Work out the finished part from the listing and answer in its coordinate system (mm). A direction names the side the tool comes from. Give positions to 0.01 mm unless a question says otherwise; leave off trailing zeros. Order: outer loops, then holes, each group sorted by start corner. A loop starts at its lowest first (then second) coordinate and runs counter-clockwise, first axis right, second up. Notation, with made-up numbers: (7.5, 20.25) -> (57.5, 20.25) arc R34 cw to (57.5, 54.25) -> close; hole circle Ø11 at (-27, 74). An arc over 180 degrees is marked (long way). Use a Markdown table: item, result. Add a question column.
```python
from build123d import *

# Parameters (mm, degrees)
BASIC_SHAPE_SKETCH_R                = 49
BASIC_SHAPE_SKETCH_R_2              = 22.5
BASIC_SHAPE_DEPTH                   = 68.03
SLIT_DEPTH                          = 98.108603635
BATTERY_SLOT_SKETCH_R               = 9.65
BATTERY_SLOT_DEPTH                  = 67.03
PATTERN_BATTERY_SLOT_COUNT          = 5
PATTERN_BATTERY_SLOT_ANGLE          = 130.88
MIRROR_BATTERY_SLOT_COPY_1_SKETCH_R = 9.65
MIRROR_BATTERY_SLOT_COPY_1_DEPTH    = 67.03
MIRROR_BATTERY_SLOT_COPY_2_SKETCH_R = 9.65
MIRROR_BATTERY_SLOT_COPY_2_DEPTH    = 67.03
MIRROR_BATTERY_SLOT_COPY_3_SKETCH_R = 9.65
MIRROR_BATTERY_SLOT_COPY_3_DEPTH    = 67.03
MIRROR_BATTERY_SLOT_COPY_4_SKETCH_R = 9.65
MIRROR_BATTERY_SLOT_COPY_4_DEPTH    = 67.03
BUS_SLIT_DEPTH                      = 67.03
CAP_INNER_LIP_DEPTH                 = 4.8
CAP_OUTER_LIP_DEPTH                 = 4.8
WIRE_SLITS_DEPTH                    = 98.108603635
WIRE_SLITS_DEPTH_BACK               = 67.03
PENNY_HOLE_SKETCH_R                 = 9.65
PENNY_HOLE_DEPTH                    = 100.807559333


with BuildPart() as part:
    # Basic_Shape_Sketch → Basic_Shape (new body)
    with BuildSketch(Plane.XY):
        Circle(BASIC_SHAPE_SKETCH_R)
        Circle(BASIC_SHAPE_SKETCH_R_2, mode=Mode.SUBTRACT)
    extrude(amount=BASIC_SHAPE_DEPTH)

    # Slit_Sketch → Slit (cut, through all)
    with BuildSketch(Plane.XY.offset(68.03)):
        with BuildLine():
            Line((-8.33, 48.286759055), (-8.33, 20.901222452))
            Line((-8.33, 20.901222452), (8.33, 20.901222452))
            Line((8.33, 20.901222452), (8.33, 48.286759055))
            ThreePointArc((8.33, 48.286759055), (0, 56.616759055), (-8.33, 48.286759055))
        make_face()
    extrude(amount=-SLIT_DEPTH, mode=Mode.SUBTRACT)

    # Battery_Slot_Sketch → Battery_Slot (cut)
    with BuildSketch(Plane.XY.offset(68.03)):
        with Locations((-10.069761866, -34.302512969)):
            Circle(BATTERY_SLOT_SKETCH_R)
    battery_slot = extrude(amount=-BATTERY_SLOT_DEPTH, mode=Mode.SUBTRACT)

    # Pattern_Battery_Slot: Battery_Slot ×5 about axis
    pattern_battery_slot_axis = Axis((0, 0, 0), (0, 0, -1))
    for i in range(1, PATTERN_BATTERY_SLOT_COUNT):
        add(battery_slot.rotate(pattern_battery_slot_axis, i * PATTERN_BATTERY_SLOT_ANGLE / (PATTERN_BATTERY_SLOT_COUNT - 1)), mode=Mode.SUBTRACT)

    # Mirror_Battery_Slot: Battery_Slot across plane
    add(battery_slot.mirror(Plane(origin=(0, 0, 0), x_dir=(0, 0, 1), z_dir=(1, 0, 0))), mode=Mode.SUBTRACT)

    # Mirror_Battery_Slot copy 1 sketch → Mirror_Battery_Slot copy 1 (cut)
    with BuildSketch(Plane(origin=(0, 0, 68.03), x_dir=(-0.8413221512344797, -0.5405340302350882, 0), z_dir=(0, 0, 1))):
        with Locations((-10.069761866, 34.302512969)):
            Circle(MIRROR_BATTERY_SLOT_COPY_1_SKETCH_R)
    extrude(amount=-MIRROR_BATTERY_SLOT_COPY_1_DEPTH, mode=Mode.SUBTRACT)

    # Mirror_Battery_Slot copy 2 sketch → Mirror_Battery_Slot copy 2 (cut)
    with BuildSketch(Plane(origin=(0, 0, 68.03), x_dir=(-0.4156459243156256, -0.9095265062656553, 0), z_dir=(0, 0, 1))):
        with Locations((-10.069761866, 34.302512969)):
            Circle(MIRROR_BATTERY_SLOT_COPY_2_SKETCH_R)
    extrude(amount=-MIRROR_BATTERY_SLOT_COPY_2_DEPTH, mode=Mode.SUBTRACT)

    # Mirror_Battery_Slot copy 3 sketch → Mirror_Battery_Slot copy 3 (cut)
    with BuildSketch(Plane(origin=(0, 0, 68.03), x_dir=(0.14193790484034807, -0.9898755634773152, 0), z_dir=(0, 0, 1))):
        with Locations((-10.069761866, 34.302512969)):
            Circle(MIRROR_BATTERY_SLOT_COPY_3_SKETCH_R)
    extrude(amount=-MIRROR_BATTERY_SLOT_COPY_3_DEPTH, mode=Mode.SUBTRACT)

    # Mirror_Battery_Slot copy 4 sketch → Mirror_Battery_Slot copy 4 (cut)
    with BuildSketch(Plane(origin=(0, 0, 68.03), x_dir=(0.6544769311996185, -0.7560819707726999, 0), z_dir=(0, 0, 1))):
        with Locations((-10.069761866, 34.302512969)):
            Circle(MIRROR_BATTERY_SLOT_COPY_4_SKETCH_R)
    extrude(amount=-MIRROR_BATTERY_SLOT_COPY_4_DEPTH, mode=Mode.SUBTRACT)

    # Bus_Slit_Sketch → Bus_Slit (cut)
    with BuildSketch(Plane.XY.offset(68.03)):
        with BuildLine():
            ThreePointArc((-9.754463235, 31.132636766), (0, -32.625), (9.754463235, 31.132636766))
            ThreePointArc((9.754463235, 31.132636766), (10.629095474, 34.20551129), (12.459123069, 36.824392423))
            ThreePointArc((12.459123069, 36.824392423), (0, -38.875), (-12.459123069, 36.824392423))
            ThreePointArc((-12.459123069, 36.824392423), (-10.629095474, 34.20551129), (-9.754463235, 31.132636766))
        make_face()
    extrude(amount=-BUS_SLIT_DEPTH, mode=Mode.SUBTRACT)

    # Cap_Inner_Lip_Sketch → Cap_Inner_Lip (add)
    with BuildSketch(Plane.XY.offset(68.03)):
        with BuildLine():
            Line((-8.33, 23.040423173), (-8.33, 20.901222452))
            ThreePointArc((-8.33, 20.901222452), (0, -22.5), (8.33, 20.901222452))
            Line((8.33, 20.901222452), (8.33, 23.040423173))
            ThreePointArc((8.33, 23.040423173), (0, -24.5), (-8.33, 23.040423173))
        make_face()
    extrude(amount=CAP_INNER_LIP_DEPTH)

    # Cap_Outer_Lip_Sketch → Cap_Outer_Lip (add)
    with BuildSketch(Plane.XY.offset(68.03)):
        with BuildLine():
            Line((-8.33, 48.286759055), (-8.33, 46.255930431))
            ThreePointArc((-8.33, 46.255930431), (0, -47), (8.33, 46.255930431))
            Line((8.33, 46.255930431), (8.33, 48.286759055))
            ThreePointArc((8.33, 48.286759055), (0, -49), (-8.33, 48.286759055))
        make_face()
    extrude(amount=CAP_OUTER_LIP_DEPTH)

    # Wire_Slits_Sketch → Wire_Slits (cut, two sides: drawn at the far end of the back side and taken through both)
    with BuildSketch(Plane.XY.offset(68.03).offset(-WIRE_SLITS_DEPTH_BACK)):
        with BuildLine():
            Line((-34.213144669, 0.12145741), (-17.213144669, 2.571194832))
            ThreePointArc((-17.213144669, 2.571194832), (-11.551118845, -1.664541654), (-15.786855331, -7.326567477))
            Line((-15.786855331, -7.326567477), (-32.786855331, -9.776304899))
            ThreePointArc((-32.786855331, -9.776304899), (-38.448881155, -5.540568413), (-34.213144669, 0.12145741))
        make_face()
        with BuildLine():
            Line((34.213144669, 0.12145741), (17.213144669, 2.571194832))
            ThreePointArc((17.213144669, 2.571194832), (11.551118845, -1.664541654), (15.786855331, -7.326567477))
            Line((15.786855331, -7.326567477), (32.786855331, -9.776304899))
            ThreePointArc((32.786855331, -9.776304899), (38.448881155, -5.540568413), (34.213144669, 0.12145741))
        make_face()
    extrude(amount=WIRE_SLITS_DEPTH + WIRE_SLITS_DEPTH_BACK, mode=Mode.SUBTRACT)

    # Penny Hole Sketch → Penny Hole (cut, through all)
    with BuildSketch(Plane.XY.offset(1)):
        with Locations((-17.602674332, 27.355927262)):
            Circle(PENNY_HOLE_SKETCH_R)
    penny_hole = extrude(amount=-PENNY_HOLE_DEPTH, mode=Mode.SUBTRACT)

    # Penny Hole Mirror: Penny Hole across plane
    add(penny_hole.mirror(Plane(origin=(0, 0, 0), x_dir=(0, 0, 1), z_dir=(1, 0, 0))), mode=Mode.SUBTRACT)


solid = part.part
```
1) The part is cut by section C-C, the plane y = -1.5. Determine the outline of the cut face in (x, z).
2) The part is cut by section B-B, the plane y = -36. Determine the outline of the cut face in (x, z), then the cut area to 3 significant figures.
3) The part is cut by section A-A, the plane y = 14.5. Determine the outline of the cut face in (x, z).
4) Flat-ended cylindrical pins translate along their axes: pin 1 (6 mm diameter, centred on y = -7.5, z = 49, fed in from -X); pin 2 (1.5 mm diameter, centred on x = -4, z = 60, fed in from -Y); pin 3 (1 mm diameter, centred on x = 24, z = 63, fed in from +Y); pin 4 (8 mm diameter, centred on x = -16.5, y = 27.5, fed in from -Z). Find the tip coordinate at first contact, or state that the pin passes through.
5) Which of the six approach directions +Z, -Z, +X, -X, +Y, -Y give full straight-line access (tool end or side, diameter ignored) to faces 1 (the flat face through (-8.33, 35, 36)), 2 (the cylindrical face through (12.96, -43.51, 34.98))?
6) Straight lines are drawn through the part: line 1 (Y direction, x = 0, z = 69); line 2 (Y direction, x = 11.5, z = 41.5); line 3 (X direction, y = 0, z = 69.6). For each, find the intervals that lie inside material, in ascending order.
A:
| question | item | result |
|---|---|---|
| 1 | outline | (-48.98, 0) -> (-22.45, 0) -> (-22.45, 1) -> (-44.34, 1) -> (-44.34, 68.03) -> (-46.98, 68.03) -> (-46.98, 72.83) -> (-48.98, 72.83) -> close; (22.45, 0) -> (48.98, 0) -> (48.98, 72.83) -> (46.98, 72.83) -> (46.98, 68.03) -> (44.34, 68.03) -> (44.34, 1) -> (22.45, 1) -> close |
| 2 | outline | (-33.24, 0) -> (33.24, 0) -> (33.24, 72.83) -> (30.22, 72.83) -> (30.22, 68.03) -> (19.57, 68.03) -> (19.57, 1) -> (-19.57, 1) -> (-19.57, 68.03) -> (-30.22, 68.03) -> (-30.22, 72.83) -> (-33.24, 72.83) -> close |
| 2 | area | 1,930 mm^2 |
| 3 | outline | (-46.81, 0) -> (-17.2, 0) -> (-17.2, 72.83) -> (-19.75, 72.83) -> (-19.75, 68.03) -> (-22.88, 68.03) -> (-22.88, 1) -> (-42.17, 1) -> (-42.17, 68.03) -> (-44.71, 68.03) -> (-44.71, 72.83) -> (-46.81, 72.83) -> close; (17.2, 0) -> (46.81, 0) -> (46.81, 72.83) -> (44.71, 72.83) -> (44.71, 68.03) -> (42.17, 68.03) -> (42.17, 1) -> (22.88, 1) -> (22.88, 68.03) -> (19.75, 68.03) -> (19.75, 72.83) -> (17.2, 72.83) -> close |
| 4 | pin 1 | x = -48.79 |
| 4 | pin 2 | y = -48.89 |
| 4 | pin 3 | y = 43 |
| 4 | pin 4 | through |
| 5 | face 1 | +Z, -Z, +Y |
| 5 | face 2 | +Z |
| 6 | line 1 | -49 to -47, -24.5 to -22.5 |
| 6 | line 2 | -47.63 to -43.85, -24.76 to -19.34, 19.34 to 24.44, 35.68 to 47.63 |
| 6 | line 3 | -49 to -47, 47 to 49 |
